Read the model definition and answer for the solid it produces. Units are mm, in the model's axes. Face numbers are marked on the shaded views. A direction names the side the tool comes from. Coordinates: 2 decimals unless noted, no trailing zeros. Loops run counter-clockwise (first coordinate to the right, second up) from the corner with the lowest first, then second, coordinate; pieces in that order, holes last. Notation, with made-up numbers: (49, -12) -> (53, -12) arc R29 cw to (53, 11) -> close; hole circle Ø8 at (24, 39). An arc over 180 degrees is marked (long way). Answer as a JSON object with one key per item and string values. Group by question number.
Q1. For the marked faces 1, 2, 3 and 4, determine the directions among +Z, -Z, +X, -X, +Y, -Y from which every point of the face is accessible in a straight line to the end or side of a thin tool.
Q2. The part is cut by section A-A on x = 0. Write down the section's boundary in (y, z) (3 decimals).
Q3. The part is cut by section B-B on y = 0. Write down the section's boundary in (x, z) (3 decimals), and give its area (3 significant figures).
Q4. Determine the mould class of the marked faces 5, 6 and 7 for opening direction X: released by +X, released by -X, zero draft, split by the parting line, or undercut.
Q5. The part is cut by section C-C on z = 40.5. Write down the section's boundary in (x, y).
Q6. Each of these flat-tipped pins is pushed along its axis until it touches: P1, Ø3, axis at x = -2, y = 12, coming from the +Z side; P2, Ø6, axis at y = 5, z = 9.5, coming from the +X side; P3, Ø5, axis at x = 3, z = 5, coming from the +Y side. Where does it stop, or does it pass through?
Q7. Straight lines are drawn through the part: line 1 along Y through (x, z) = (0, 9) (3 decimals); line 2 along Z through (x, y) = (-13.5, 6.5). For each, find the intervals that lie inside material, in ascending order. Write a range as [from, to].
Q8. The part is cut by section D-D on x = -6.5. Write down the section's boundary in (y, z).
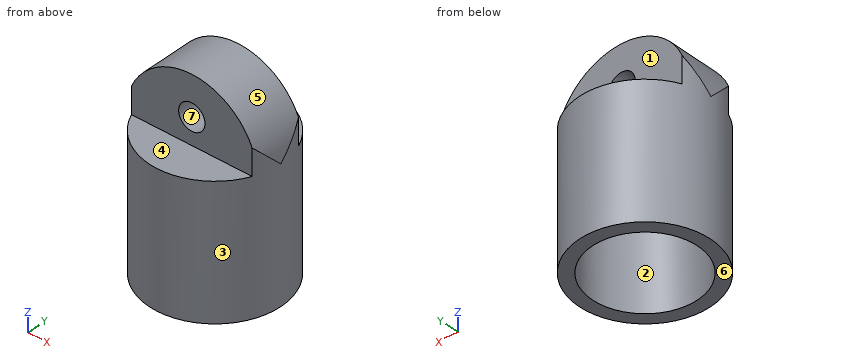
from build123d import *

# Parameters (mm, degrees)
F0_R          = 15.875
F1_DEPTH      = 31.75
F2_R          = 12.7
F3_DEPTH      = 25.4
F4_R          = 3.175
F5_DEPTH      = 6.35
F5_DEPTH_BACK = 6.35
F6_W          = 11.146276543
F6_H          = 50.8


# Not quite as in the source:
# - after a boolean that leaves OpenCascade's solid faulty, fix() repairs it


with BuildPart() as f1:
    # F0 (on Top) → F1 (new body)
    with BuildSketch(Plane.XY):
        Circle(F0_R)
    extrude(amount=F1_DEPTH)

    # F2 (on face) → F3 (cut)
    with BuildSketch(Plane(origin=(0, 0, 0), x_dir=(1, 0, 0), z_dir=(0, 0, -1))):
        Circle(F2_R)
    extrude(amount=-F3_DEPTH, mode=Mode.SUBTRACT)

    # F4 (on Front) → F5 (join, two sides)
    with BuildSketch(Plane.XZ) as f5_sk:
        with BuildLine():
            ThreePointArc((15.875, 31.75), (0, 47.625), (-15.875, 31.75))
            Line((-15.875, 31.75), (15.875, 31.75))
        make_face()
        with Locations((0, 38.1)):
            Circle(F4_R, mode=Mode.SUBTRACT)
    extrude(amount=F5_DEPTH)
    extrude(f5_sk.sketch, amount=-F5_DEPTH_BACK)

    # F6 (on Front) → F7 (revolve, cut)
    with BuildSketch(Plane.XZ):
        with Locations((-21.4481382715, 25.4)):
            Rectangle(F6_W, F6_H)
    revolve(axis=Axis((0, 0, 12.5730000436), (0, 0, 1)), mode=Mode.SUBTRACT)

    add(f1.part.fix(), mode=Mode.REPLACE)


solid = f1.part
Final values:
{
 "1": {"face 1": "+Z, +X, -X, +Y", "face 2": "-Z", "face 3": "+Z, -Z", "face 4": "+Z, +X, -X, -Y"},
 "2": {"outline": "(-15.875, 0) -> (-12.7, 0) -> (-12.7, 25.4) -> (12.7, 25.4) -> (12.7, 0) -> (15.875, 0) -> (15.875, 31.75) -> (6.35, 31.75) -> (6.35, 34.925) -> (-6.35, 34.925) -> (-6.35, 31.75) -> (-15.875, 31.75) -> close; (-6.35, 41.275) -> (6.35, 41.275) -> (6.35, 47.625) -> (-6.35, 47.625) -> close"},
 "3": {"outline": "(-15.875, 0) -> (-12.7, 0) -> (-12.7, 25.4) -> (12.7, 25.4) -> (12.7, 0) -> (15.875, 0) -> (15.875, 31.75) arc R15.875 ccw to (-15.875, 31.75) -> close; hole circle Ø6.35 at (0, 38.1)", "area": "727 mm2"},
 "4": {"face 5": "split by the parting line", "face 6": "zero draft", "face 7": "undercut"},
 "5": {"outline": "(-13.25, -6.35) -> (-2.08, -6.35) -> (-2.08, 6.35) -> (-13.25, 6.35) -> close; (2.08, -6.35) -> (13.25, -6.35) -> (13.25, 6.35) -> (2.08, 6.35) -> close"},
 "6": {"P1": "stops at z = 31.75", "P2": "stops at x = 15.75", "P3": "stops at y = 15.87"},
 "7": {"line 1": "y = [-15.875, -12.7], [12.7, 15.875]", "line 2": "z = [0, 31.75]"},
 "8": {"outline": "(-14.48, 0) -> (-10.91, 0) -> (-10.91, 25.4) -> (10.91, 25.4) -> (10.91, 0) -> (14.48, 0) -> (14.48, 31.75) -> (6.35, 31.75) -> (6.35, 46.23) -> (-6.35, 46.23) -> (-6.35, 31.75) -> (-14.48, 31.75) -> close"}
}
